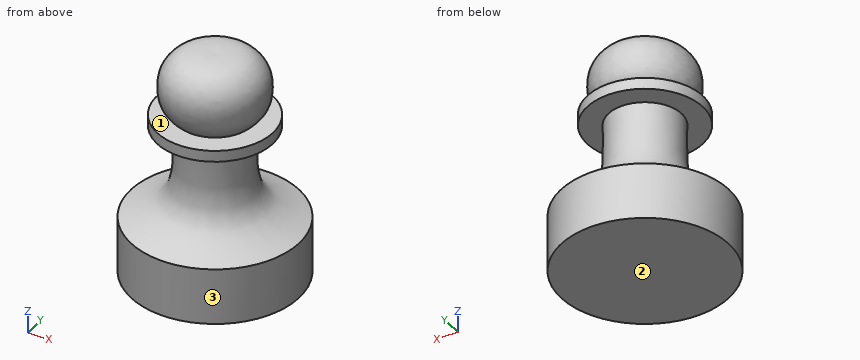
```python
from build123d import *


with BuildPart() as f1:
    # F0 (on Front) → F1 (revolve)
    with BuildSketch(Plane.XZ):
        Polygon((0, 36.456387707), (0, 33.916387707), (8.3032539114, 33.916387707), (13.1206531078, 33.916387707), (13.1206531078, 36.456387707), (8.3377687261, 36.456387707), align=None)
        with BuildLine():
            Line((0, 33.916387707), (0, 0))
            Line((0, 0), (19.05, 0))
            Line((19.05, 0), (19.05, 12.7))
            add(Edge.make_bspline(
                [(19.05, 12.7), (15.6836506907, 14.0721710831), (9.3393919334, 16.6581797265), (8.0395309284, 25.3025272106), (8.2135911581, 30.9877751162), (8.3032539114, 33.916387707)],
                knots=[0, 0, 0, 0, 0.3540562683, 0.6672583189, 1, 1, 1, 1], degree=3))
            Line((8.3032539114, 33.916387707), (0, 33.916387707))
        make_face()
        with BuildLine():
            Line((0, 50.8), (0, 36.456387707))
            Line((0, 36.456387707), (8.3377687261, 36.456387707))
            add(Edge.make_bspline(
                [(8.3377687261, 36.456387707), (10.3048640053, 38.2170454213), (11.3878356839, 40.544651372), (11.392239415, 46.1874953748), (8.3974127327, 49.5973153016), (5.2773343635, 50.7991233773), (1.7471459357, 50.9378901576), (0, 50.8)],
                knots=[0, 0, 0, 0, 0.2154525637, 0.4253980018, 0.6169348664, 0.7858471635, 1, 1, 1, 1], degree=3))
        make_face()
    revolve(axis=Axis((0, 0, 25.4), (0, 0, 1)))


solid = f1.part
```
Can you work these out from the model? Positions are in its coordinate system, mm. Face numbers are marked on the shaded views. Give positions to 0.01 mm unless a question says otherwise; leave off trailing zeros. Write each loop counter-clockwise with the first axis right and the second up, starting at its lowest first coordinate (ties: lowest second). Pieces come first, ordered by that corner, then holes. Notation, with made-up numbers: (12.25, 42) -> (71.25, 42) arc R21 cw to (71.25, 67) -> close; hole circle Ø8 at (-4.5, 81). An arc over 180 degrees is marked (long way). One line per item, written item: value.
Q1. Please list where these lines run through material, in increasing order: line 1 (Z direction, x = -6.5, y = -8.5); line 2 (Z direction, x = -5, y = 10.5); line 3 (Z direction, x = -7, y = -8). Write a range as [from, to].
Results found:
line 1: z = [0, 17.47], [33.92, 36.46], [39.45, 46.3]
line 2: z = [0, 16.56], [33.92, 36.46]
line 3: z = [0, 17.55], [33.92, 36.46], [39.29, 46.46]
Q2. Imagine slicing it at A-A on z = 7. Please give me the cut outline in (x, y).
Results found:
outline: circle Ø38.1 at (0, 0)
Q3. For P1, Ø2, axis at x = -10.5, z = 34, coming from the +Y side; P2, Ø1.5, axis at y = -8.5, z = 33.5, coming from the +X side; P3, Ø8, axis at x = -15, z = 15, coming from the -Y side, each with a flat end and sliding along its axis, tell me the tip position at first contact or that it passes through.
Results found:
P1: stops at y = 9.05
P2: stops at x = 10.49
P3: stops at y = -15.01
Q4. We'd pull the mould along Z, two halves only. Please class the marked faces 1, 2 and 3: +Z half, -Z half, draft (parallel to the pull), parting line (faces both ways), or undercut.
Results found:
face 1: undercut
face 2: -Z half
face 3: draft
